Could you check a few things on this model? Use its own coordinates, in mm. Coordinates: 2 decimals unless noted, no trailing zeros. Write each loop counter-clockwise with the first axis right and the second up, starting at its lowest first coordinate (ties: lowest second). Pieces come first, ordered by that corner, then holes.
```python
from build123d import *

# Parameters (mm, degrees)
BASE_DEPTH         = 5.334
CUT_EXTRUDE1_REACH = 7.334
SKETCH3_W          = 25.4
SKETCH3_H          = 10.668


with BuildPart() as part:
    # Sketch1 → Base (new body)
    with BuildSketch(Plane(origin=(0, 0, 0), x_dir=(1, 0, 0), z_dir=(0, 1, 0))):
        Polygon((0, 0), (380.417035208, -21.068443786), (380.417035208, -97.633742074), (264.564463463, -117.810081629), (264.564463463, -124.160081629), (0, -170.235385513), align=None)
    extrude(amount=BASE_DEPTH)

    # Sketch3 → Cut-Extrude1 (cut, up to next)
    with BuildSketch(Plane.XZ, mode=Mode.PRIVATE) as cut_extrude1_sk1:
        with Locations((278.817035208, 59.945526857)):
            Rectangle(SKETCH3_W, SKETCH3_H)
    cut_extrude1_tool1 = extrude(cut_extrude1_sk1.sketch, amount=-CUT_EXTRUDE1_REACH, mode=Mode.PRIVATE) & part.part
    add(cut_extrude1_tool1.solids().sort_by_distance((278.817035, 0, 59.945527))[0], mode=Mode.SUBTRACT)
    # Sketch3 → Cut-Extrude1 (cut, up to next)
    with BuildSketch(Plane.XZ, mode=Mode.PRIVATE) as cut_extrude1_sk2:
        with Locations((88.9, 59.945526857)):
            Rectangle(SKETCH3_W, SKETCH3_H)
    cut_extrude1_tool2 = extrude(cut_extrude1_sk2.sketch, amount=-CUT_EXTRUDE1_REACH, mode=Mode.PRIVATE) & part.part
    add(cut_extrude1_tool2.solids().sort_by_distance((88.9, 0, 59.945527))[0], mode=Mode.SUBTRACT)


solid = part.part
```
1. Please list where these lines run through material, in increasing order: line 1 along X through (y, z) = (4.9, 120); line 2 along Z through (x, y) = (93, 4.05); line 3 along Z through (x, y) = (268, 4.8).
Verdict:
line 1: x = 0 to 264.56
line 2: z = 5.15 to 54.61, 65.28 to 154.04
line 3: z = 14.84 to 54.61, 65.28 to 117.21
2. I want a section at C-C on x = 310. Please give me the cut outline in (y, z), plus the area to 3 significant figures.
Verdict:
outline: (0, 17.17) - (5.33, 17.17) - (5.33, 109.9) - (0, 109.9) - close
area: 495 mm2
3. I want a section at D-D on z = 147. Please give me the cut outline in (x, y), plus the area to 3 significant figures.
Verdict:
outline: (0, 0) - (133.42, 0) - (133.42, 5.33) - (0, 5.33) - close
area: 712 mm2
4. I want a section at A-A on z = 59.5. Please give me the cut outline in (x, y).
Verdict:
outline: (0, 0) - (76.2, 0) - (76.2, 5.33) - (0, 5.33) - close; (101.6, 0) - (266.12, 0) - (266.12, 5.33) - (101.6, 5.33) - close; (291.52, 0) - (380.42, 0) - (380.42, 5.33) - (291.52, 5.33) - close
5. I want a section at B-B on y = 3.4. Please give me the cut outline in (x, z).
Verdict:
outline: (0, 0) - (380.42, 21.07) - (380.42, 97.63) - (264.56, 117.81) - (264.56, 124.16) - (0, 170.24) - close; hole (76.2, 54.61) - (101.6, 54.61) - (101.6, 65.28) - (76.2, 65.28) - close; hole (266.12, 54.61) - (291.52, 54.61) - (291.52, 65.28) - (266.12, 65.28) - close
6. For pin 1 (1.6 mm diameter, centred on x = 91, y = 2, fed in from +Z); pin 2 (1.6 mm diameter, centred on x = 275, y = 2, fed in from -Z); pin 3 (1.5 mm diameter, centred on x = 81, y = 3.5, fed in from -Z), each with a flat end and sliding along its axis, tell me the tip position at first contact or that it passes through.
Verdict:
pin 1: stops at z = 154.53
pin 2: stops at z = 15.19
pin 3: stops at z = 4.44
